The drawing under review shows one solid part. Ordinate dimensions are in mm from its lowest x, y, z. Round coordinates to 2 decimals unless told otherwise and drop trailing zeros. Loops run counter-clockwise (first coordinate to the right, second up) from the corner with the lowest first, then second, coordinate; pieces in that order, holes last. Notation, with made-up numbers: (-12, 2) -> (29, 2) arc R14 cw to (29, 11) -> close; hole circle Ø3 at (65, 40). An arc over 180 degrees is marked (long way). Use a Markdown table: item, result. Add a question column.
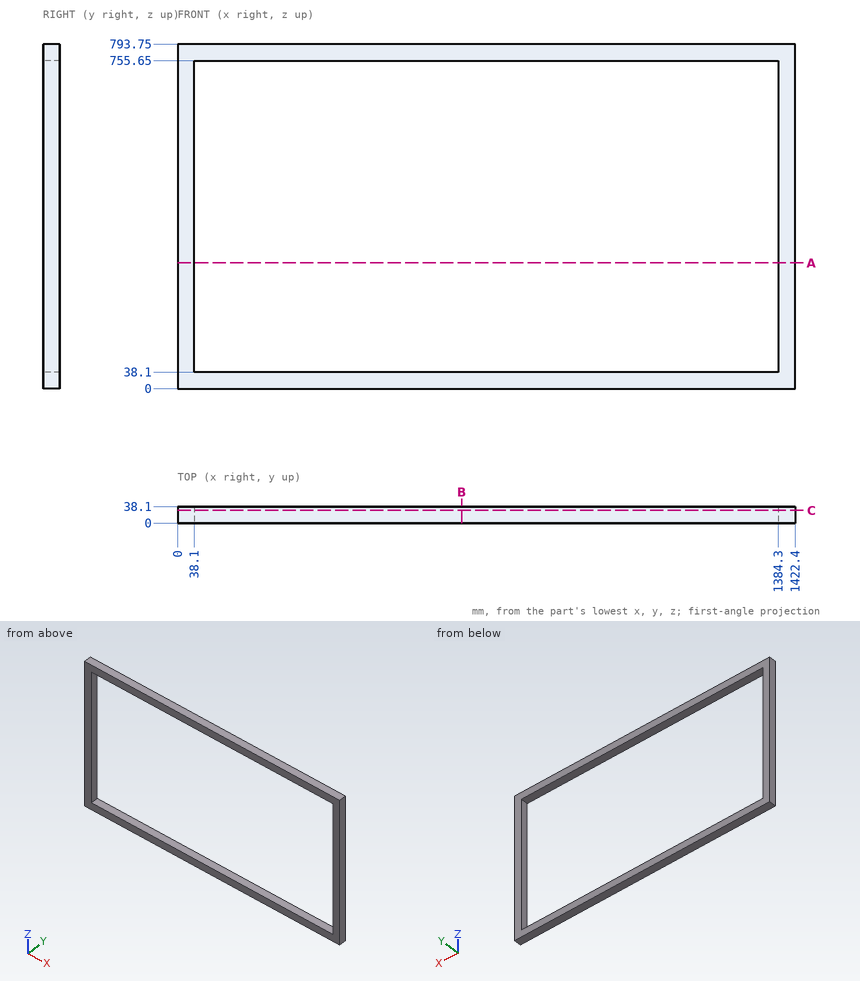
1. To check wall thickness, follow probe 1 along X at (y, z) = (10.5, 556.5); probe 2 along Z at (x, y) = (1265.5, 23.5). State the ranges of each line that lie inside material, in increasing order. Write a range as from..to.
2. Consider section A-A on z = 289.5. State the section outline as (x, y) points.
3. Consider section B-B on x = 654.5. State the section outline as (y, z) points.
4. Consider section C-C on y = 29.5. State the section outline as (x, z) points, plus the area to 3 significant figures.
Verdict:
| question | item | result |
|---|---|---|
| 1 | probe 1 | x = 0..38.1, 1384.3..1422.4 |
| 1 | probe 2 | z = 0..38.1, 755.65..793.75 |
| 2 | outline | (0, 0) -> (38.1, 0) -> (38.1, 38.1) -> (0, 38.1) -> close; (1384.3, 0) -> (1422.4, 0) -> (1422.4, 38.1) -> (1384.3, 38.1) -> close |
| 3 | outline | (0, 0) -> (38.1, 0) -> (38.1, 38.1) -> (0, 38.1) -> close; (0, 755.65) -> (38.1, 755.65) -> (38.1, 793.75) -> (0, 793.75) -> close |
| 4 | outline | (0, 0) -> (1422.4, 0) -> (1422.4, 793.75) -> (0, 793.75) -> close; hole (38.1, 38.1) -> (1384.3, 38.1) -> (1384.3, 755.65) -> (38.1, 755.65) -> close |
| 4 | area | 163,000 mm² |
